```python
from build123d import *

# Parameters (mm, degrees)
F3_D     = 5.2
F5_D     = 8
F5_DEPTH = 28.401


with BuildPart() as f1:
    # F0 (on Front) → F1 (revolve)
    with BuildSketch(Plane.XZ):
        Polygon((-32.6399943951, 7.8358277731), (-32.6399943951, -12.5641722269), (-6.2399943951, -12.5641722269), (-6.2399943951, -2.0641722269), (-26.6399943951, -2.0641722269), (-26.6399943951, 7.8358277731), align=None)
    revolve(axis=Axis((0, 0, -20.5641722269), (-1, 0, 0)))

    # F3 (through all)
    with Locations(Plane.YZ.offset(-26.6399943951)):
        with Locations((-11.4125286283, 0), (12.1028312422, -0.3985464), (23.5153598705, -20.9627186269), (11.4125286283, -41.1283444539), (-12.1028312422, -40.7297980539), (-23.5153598705, -20.165625827)):
            Hole(F3_D / 2)

    # F5 (through all, one way)
    with BuildSketch(Plane.XZ):
        with Locations((-16.4399943951, -22.3195198923)):
            Circle(F5_D / 2)
    extrude(amount=-F5_DEPTH, mode=Mode.SUBTRACT)


solid = f1.part
```
For this review, take the finished solid that the model builds, in its own axes (mm). A direction names the side the tool comes from. Give positions to 0.01 mm unless a question says otherwise; leave off trailing zeros. Write each loop counter-clockwise with the first axis right and the second up, starting at its lowest first coordinate (ties: lowest second). Pieces come first, ordered by that corner, then holes.
Item 1: Wall thickness on probe 1 along Z at (x, y) = (-30.5, 2); probe 2 along Z at (x, y) = (-27.75, -4); probe 3 along X at (y, z) = (19, -6.5): over which ranges is each line inside the solid? List them lowest first.
Item 2: Take a section at D-D (x = -21.5). Give the boundary of the cut face in (y, z).
Item 3: Insertion check: P1, Ø8, axis at x = -21.5, z = 0.5, coming from the -Y side; P2, Ø6, axis at y = -11.41, z = 0, coming from the +X side; P3, Ø10, axis at x = -24.5, z = -14, coming from the -Y side. Each pin has a flat end and moves straight along its axis. Give the tip position at first contact, or say it passes through.
Item 4: Take a section at A-A (y = 0). Give the boundary of the cut face in (x, z), and give its area (3 significant figures).
Item 5: The part is to be moulded in two halves that separate along Z. For faces 1 (the face through (-29.682, 1.249, -48.937)), 2 (the face through (-29.68, 22.32, -23.27)), 3 (the face through (-26.64, -19, -20)), say which applies: +Z half, -Z half, draft (parallel to the pull), parting line (faces both ways), or undercut.
Item 6: Machinability: for faces 4 (the face through (-16.6, -16.4, -12)), 5 (the face through (-32.64, -6, -15)), 6 (the face through (-14.594, 13.377, -25.868)), which of the approach directions +Z, -Z, +X, -X, +Y, -Y give a long, thin tool a straight path to every point of the face, cutting with its end or side? Answer none if there is none.
Item 7: Take a section at C-C (x = -30.5). Give the boundary of the cut face in (y, z), and give its area (3 significant figures).
Item 8: Take a section at B-B (z = -27). Give the boundary of the cut face in (x, y).
Established:
1. probe 1: z = -48.89 to -28.31, -12.82 to 7.77
1. probe 2: z = -48.68 to -27.49, -13.64 to 7.55
1. probe 3: x = -32.64 to -26.64
2. outline: circle Ø37 at (0, -20.56); hole circle Ø16 at (0, -20.56)
3. P1: stops at y = -7.15
3. P2: stops at x = -26.64
3. P3: stops at y = -28.33
4. outline: (-32.64, -48.96) - (-26.64, -48.96) - (-26.64, -39.06) - (-6.24, -39.06) - (-6.24, -28.56) - (-32.64, -28.56) - close; (-32.64, -12.56) - (-6.24, -12.56) - (-6.24, -2.06) - (-26.64, -2.06) - (-26.64, 7.84) - (-32.64, 7.84) - close
4. area: 673 mm2
5. face 1: parting line
5. face 2: undercut
5. face 3: draft
6. face 4: +X
6. face 5: +Z, -Z, -X, +Y, -Y
6. face 6: +Y
7. outline: circle Ø56.8 at (0, -20.56); hole circle Ø5.2 at (-23.52, -20.17); hole circle Ø5.2 at (-12.1, -40.73); hole circle Ø5.2 at (-11.41, 0); hole circle Ø16 at (0, -20.56); hole circle Ø5.2 at (11.41, -41.13); hole circle Ø5.2 at (12.1, -0.4); hole circle Ø5.2 at (23.52, -20.96)
7. area: 2,210 mm2
8. outline: (-32.64, -27.66) - (-26.64, -27.66) - (-26.64, -17.34) - (-6.24, -17.34) - (-6.24, -4.75) - (-32.64, -4.75) - close; (-32.64, 4.75) - (-6.24, 4.75) - (-6.24, 17.34) - (-26.64, 17.34) - (-26.64, 27.66) - (-32.64, 27.66) - close
